Design review of the part built by this model. Coordinates are the model's own, in mm. A direction names the side the tool comes from. Round coordinates to 2 decimals unless told otherwise and drop trailing zeros. Order: outer loops, then holes, each group sorted by start corner. A loop starts at its lowest first (then second) coordinate and runs counter-clockwise, first axis right, second up. Notation, with made-up numbers: M 21.25,53.5 L 39.25,53.5 A15 cw 39.25,58.5 Z; hole C 42.5,83.25 d3. An arc over 180 degrees is marked long. Write each question's results on one line, items separated by ' | '. Start each with the question number.
Item 1: Take a section at C-C, the plane y = -0.5. Write out the cut boundary in (x, z).
Item 2: Clearance check with flat-ended pins moving along their axes: pin 1 (5.5 mm diameter, centred on x = -0.5, y = -1.5, fed in from +Z); pin 2 (3.5 mm diameter, centred on x = 0, y = 0, fed in from +Z); pin 3 (5.5 mm diameter, centred on y = -1.5, z = 6.5, fed in from +X). State where each tip first meets the part, or that it passes through.
Item 3: Take a section at A-A, the plane z = 6.55. Write out the cut boundary in (x, y) (3 decimals).
Item 4: Machinability: for faces 4 (the flat face through (-7, 3.525, 7)), 5 (the flat face through (-5, 5.525, 2)), 6 (the cylindrical face through (2.1, 0.66, -2.74)), 7 (the flat face through (-0.34, -2.53, 6.09)), 8 (the flat face through (1, 0, 1.75)), which of the approach directions +Z, -Z, +X, -X, +Y, -Y give a long, thin tool a straight path to every point of the face, cutting with its end or side? Answer none if there is none.
Item 5: The part is to be moulded in two halves that separate along X. For faces 1 (the flat face through (-7, -3.525, 8)), 2 (the cylindrical face through (-9.29, -0.29, 8.73)), 3 (the flat face through (-3.038, 1.787, 0.024)), say which applies: +X half, -X half, draft (parallel to the pull), parting line (faces both ways), or undercut.
Item 6: Take a section at D-D, the plane x = -8. Write out the cut boundary in (y, z) (3 decimals).
Item 7: Wall thickness on line 1 (Z direction, x = -8.65, y = 0); line 2 (Y direction, x = -2.25, z = 6.55) (3 decimals); line 3 (Z direction, x = -9.8, y = 0): over which ranges is each line inside the solid? List them lowest first. Write a range as [from, to].
Item 8: Take a section at B-B, the plane x = 3.25. Write out the cut boundary in (y, z) (3 decimals).
```python
from build123d import *

# Parameters (mm, degrees)
PAD_DEPTH         = 1.75
PAD001_DEPTH      = 1.75
PAD002_DEPTH      = 5.525
SKETCH003_R       = 2.2
POCKET_DEPTH      = 2.001
POCKET_DEPTH_BACK = -12.301
SKETCH004_R       = 2.2
POCKET001_DEPTH   = 2.001


with BuildPart() as pad:
    # Sketch → Pad (new body, symmetric)
    with BuildSketch(Plane.XY):
        Polygon((2.03516, 3.525), (-2.03516, 3.525), (-4.070319, 0), (-2.03516, -3.525), (2.03516, -3.525), (4.070319, -3.525), (4.070319, 3.525), align=None)
    extrude(amount=PAD_DEPTH, both=True)


with BuildPart() as pad001:
    # Sketch001 → Pad001 (new body, symmetric)
    with BuildSketch(Plane.YZ.offset(-6.55)):
        Polygon((0, 2.479681), (3.525, 4.51484), (3.525, 8.58516), (3.525, 10.620319), (-3.525, 10.620319), (-3.525, 8.58516), (-3.525, 4.51484), align=None)
    extrude(amount=PAD001_DEPTH, both=True)


with BuildPart() as pocket001:
    # Sketch002 → Pad002 (new body, symmetric)
    with BuildSketch(Plane.XZ):
        Polygon((-10.3, 10.55), (-10.3, -3.042893), (-9.592893, -3.75), (4, -3.75), (4, 1.75), (-4.8, 10.55), align=None)
    extrude(amount=PAD002_DEPTH, both=True)

    # Cut: cut Pad001
    add(pad001.part, mode=Mode.SUBTRACT)

    # Cut001: cut Pad
    add(pad.part, mode=Mode.SUBTRACT)

    # Sketch003 → Pocket (cut, two sides)
    with BuildSketch(Plane.YZ.offset(-8.3)) as pocket_sk:
        with Locations((0, 6.55)):
            Circle(SKETCH003_R)
    extrude(amount=-POCKET_DEPTH, mode=Mode.SUBTRACT)
    extrude(pocket_sk.sketch, amount=-POCKET_DEPTH_BACK, mode=Mode.SUBTRACT)

    # Sketch004 → Pocket001 (cut, through all)
    with BuildSketch(Plane.XY.offset(-1.75)):
        Circle(SKETCH004_R)
    extrude(amount=-POCKET001_DEPTH, mode=Mode.SUBTRACT)


solid = pocket001.part
```
Results list:
1) outline: M -10.3,-3.04 L -9.59,-3.75 L -2.14,-3.75 L -2.14,-1.75 L -3.78,-1.75 L -3.78,1.75 L 4,1.75 L 1.34,4.41 L -4.8,4.41 L -4.8,2.77 L -8.3,2.77 L -8.3,4.41 L -10.3,4.41 Z; M -10.3,8.69 L -8.3,8.69 L -8.3,10.55 L -10.3,10.55 Z; M -4.8,8.69 L -2.94,8.69 L -4.8,10.55 Z; M 2.14,-3.75 L 4,-3.75 L 4,-1.75 L 2.14,-1.75 Z
2) pin 1: z = 9 | pin 2: z = 5.22 | pin 3: x = 2
3) outline: M -10.3,-5.525 L -0.8,-5.525 L -0.8,-2.2 L -4.8,-2.2 L -4.8,-3.525 L -8.3,-3.525 L -8.3,-2.2 L -10.3,-2.2 Z; M -10.3,2.2 L -8.3,2.2 L -8.3,3.525 L -4.8,3.525 L -4.8,2.2 L -0.8,2.2 L -0.8,5.525 L -10.3,5.525 Z
4) face 4: +Z | face 5: +Z, -Z, +X, -X, +Y | face 6: -Z | face 7: +Z, +X, +Y, -Y | face 8: +X
5) face 1: undercut | face 2: draft | face 3: +X half
6) outline: M -5.525,-3.75 L 5.525,-3.75 L 5.525,10.55 L 3.525,10.55 L 3.525,4.515 L 0,2.48 L -3.525,4.515 L -3.525,10.55 L -5.525,10.55 Z
7) line 1: [-3.75, 4.35], [8.75, 10.55] | line 2: [-5.525, -2.2], [2.2, 5.525] | line 3: [-3.54, 4.35], [8.75, 10.55]
8) outline: M -5.525,-3.75 L 5.525,-3.75 L 5.525,2.5 L -5.525,2.5 Z; hole M -3.525,-1.75 L 3.525,-1.75 L 3.525,1.75 L -3.525,1.75 Z
